The model under review builds one solid part; all positions refer to its coordinate system, in mm. Give positions to 0.01 mm unless a question says otherwise; leave off trailing zeros. Loops run counter-clockwise (first coordinate to the right, second up) from the corner with the lowest first, then second, coordinate; pieces in that order, holes last. Notation, with made-up numbers: (-2.75, 56) -> (31.25, 56) arc R21 ccw to (31.25, 95) -> close; hole circle Ø9 at (67.5, 59). An arc over 180 degrees is marked (long way). Write each question's results on one line, items separated by ' | '. Start each with the question number.
Q1. We need section B-B (z = -5.75). Write out the cut boundary in (x, y), plus the area to 3 significant figures.
Q2. Wall thickness on L1, parallel to X at y = 4.05, z = -6.75; L2, parallel to Z at x = -99, y = 1.45; L3, parallel to X at y = 3.4, z = -15.25: over which ranges is each line inside the solid? List them lowest first. Write a range as [from, to].
Q3. We need section A-A (y = 4.55). Write out the cut boundary in (x, z).
Q4. We need section D-D (z = -20). Write out the cut boundary in (x, y).
Q5. We need section C-C (x = -81). Write out the cut boundary in (y, z).
Q6. Insertion check: pin 1 Ø1.6 at (y, z) = (2.5, -7) entering from -X; pin 2 Ø1.6 at (x, y) = (85.5, 1.5) entering from +Z; pin 3 Ø2.5 at (y, z) = (3.5, -6) entering from +X. Each pin has a flat end and moves straight along its axis. Give the tip position at first contact, or say it passes through.
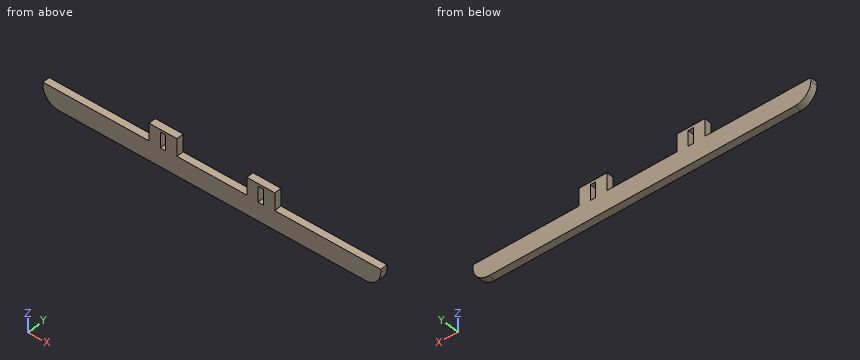
from build123d import *

# Parameters (mm, degrees)
SKETCH1_W             = 62
SKETCH1_H             = 12.7
BOSS_EXTRUDE1_DEPTH   = 5.38
SKETCH2_W             = 20.5
SKETCH2_H             = 5.38
CUT_EXTRUDE1_DEPTH    = 10.16
SKETCH3_W             = 4
SKETCH3_H             = 8.7
CUT_EXTRUDE2_DEPTH    = 5.38
SKETCH4_W             = 2.54
SKETCH4_H             = 5.38
BOSS_EXTRUDE2_DEPTH   = 59.22
SKETCH5_W             = 2.54
SKETCH5_H             = 5.38
BOSS_EXTRUDE3_DEPTH   = 11.5
BODY_MOVE_COPY3_ANGLE = 180
SKETCH6_W             = 21
SKETCH6_H             = 5.38
BOSS_EXTRUDE4_DEPTH   = 3
SKETCH7_W             = 21
SKETCH7_H             = 5.38
BOSS_EXTRUDE5_DEPTH   = 3
SKETCH8_W             = 4
SKETCH8_H             = 5.38
CUT_EXTRUDE3_DEPTH    = 3
SKETCH9_W             = 4
SKETCH9_H             = 5.38
CUT_EXTRUDE4_DEPTH    = 3
SKETCH11_W            = 253.94
SKETCH11_H            = 5.38
BOSS_EXTRUDE6_DEPTH   = 12
FILLET1_R             = 12


with BuildPart() as part:
    # Sketch1 → Boss-Extrude1 (new body)
    with BuildSketch(Plane(origin=(0, 0, 0), x_dir=(1, 0, 0), z_dir=(0, 1, 0))):
        with Locations((-31, 6.35)):
            Rectangle(SKETCH1_W, SKETCH1_H)
    extrude(amount=BOSS_EXTRUDE1_DEPTH)

    # Sketch2 → Cut-Extrude1 (cut)
    with BuildSketch(Plane.XY):
        with Locations((-51.75, 2.69)):
            Rectangle(SKETCH2_W, SKETCH2_H)
        with Locations((-10.25, 2.69)):
            Rectangle(SKETCH2_W, SKETCH2_H)
    extrude(amount=-CUT_EXTRUDE1_DEPTH, mode=Mode.SUBTRACT)

    # Sketch3 → Cut-Extrude2 (cut)
    with BuildSketch(Plane(origin=(0, 5.38, 0), x_dir=(1, 0, 0), z_dir=(0, 1, 0))):
        with Locations((-31, 6.35)):
            Rectangle(SKETCH3_W, SKETCH3_H)
    extrude(amount=-CUT_EXTRUDE2_DEPTH, mode=Mode.SUBTRACT)

    # Sketch4 → Boss-Extrude2 (add)
    with BuildSketch(Plane.ZY.offset(62)):
        with Locations((-11.43, 2.69)):
            Rectangle(SKETCH4_W, SKETCH4_H)
    extrude(amount=BOSS_EXTRUDE2_DEPTH)


with BuildPart() as body_2:
    # Body-Move/Copy1: copy of part
    add(part.part.moved(Location((0, 31.265873305, 0))))


with BuildPart() as part_1:
    add(part.part)

    # Sketch5 → Boss-Extrude3 (add)
    with BuildSketch(Plane(origin=(0, 0, 0), x_dir=(0, 0, -1), z_dir=(1, 0, 0))):
        with Locations((11.43, 2.69)):
            Rectangle(SKETCH5_W, SKETCH5_H)
    extrude(amount=BOSS_EXTRUDE3_DEPTH)


with BuildPart() as body_2_1:
    # Body-Move/Copy2: moved
    add(body_2.part.moved(Location((152.693560216, 0, 0))))


with BuildPart() as body_2_2:
    # Body-Move/Copy3: moved
    add(body_2_1.part.rotate(Axis((92.083560216, 33.955873305, 0), (0, 0, 1)), BODY_MOVE_COPY3_ANGLE))


with BuildPart() as body_2_3:
    # Body-Move/Copy4: read off the stored shape, not the designer's step
    # Body-Move/Copy4: moved
    add(body_2_2.part.moved(Location((-19.9735602, -31.2658733, 0))))

    # Combine1: union part
    add(part_1.part)

    # Sketch6 → Boss-Extrude4 (add)
    with BuildSketch(Plane.XY):
        with Locations((-31, 2.69)):
            Rectangle(SKETCH6_W, SKETCH6_H)
    extrude(amount=BOSS_EXTRUDE4_DEPTH)

    # Sketch7 → Boss-Extrude5 (add)
    with BuildSketch(Plane.XY):
        with Locations((42.5, 2.69)):
            Rectangle(SKETCH7_W, SKETCH7_H)
    extrude(amount=BOSS_EXTRUDE5_DEPTH)

    # Sketch8 → Cut-Extrude3 (cut)
    with BuildSketch(Plane(origin=(0, 0, -2), x_dir=(-1, 0, 0), z_dir=(0, 0, -1))):
        with Locations((31, 2.69)):
            Rectangle(SKETCH8_W, SKETCH8_H)
    extrude(amount=-CUT_EXTRUDE3_DEPTH, mode=Mode.SUBTRACT)

    # Sketch9 → Cut-Extrude4 (cut)
    with BuildSketch(Plane(origin=(0, 0, -2), x_dir=(-1, 0, 0), z_dir=(0, 0, -1))):
        with Locations((-42.5, 2.69)):
            Rectangle(SKETCH9_W, SKETCH9_H)
    extrude(amount=-CUT_EXTRUDE4_DEPTH, mode=Mode.SUBTRACT)

    # Sketch11 → Boss-Extrude6 (add)
    with BuildSketch(Plane(origin=(0, 0, -12.7), x_dir=(-1, 0, 0), z_dir=(0, 0, -1))):
        with Locations((-5.75, 2.69)):
            Rectangle(SKETCH11_W, SKETCH11_H)
    extrude(amount=BOSS_EXTRUDE6_DEPTH)

    # Fillet1
    fillet1_edges = [body_2_3.edges().sort_by_distance(p)[0] for p in [
        (132.72, 2.69, -24.7),
        (-121.22, 2.69, -24.7),
    ]]
    fillet(fillet1_edges, radius=FILLET1_R)


solid = body_2_3.part
Output:
1) outline: (-41.5, 0) -> (-33, 0) -> (-33, 5.38) -> (-41.5, 5.38) -> close; (-29, 0) -> (-20.5, 0) -> (-20.5, 5.38) -> (-29, 5.38) -> close; (32, 0) -> (40.5, 0) -> (40.5, 5.38) -> (32, 5.38) -> close; (44.5, 0) -> (53, 0) -> (53, 5.38) -> (44.5, 5.38) -> close | area: 183 mm2
2) L1: [-41.5, -33], [-29, -20.5], [32, 40.5], [44.5, 53] | L2: [-24.7, -10.16] | L3: [-120.95, 132.45]
3) outline: (-121.22, -12.7) arc R12 ccw to (-109.22, -24.7) -> (120.72, -24.7) arc R12 ccw to (132.72, -12.7) -> (132.72, -10.16) -> (53, -10.16) -> (53, 3) -> (32, 3) -> (32, -10.16) -> (-20.5, -10.16) -> (-20.5, 3) -> (-41.5, 3) -> (-41.5, -10.16) -> (-121.22, -10.16) -> close; hole (-33, -10.7) -> (-29, -10.7) -> (-29, 1) -> (-33, 1) -> close; hole (40.5, -10.7) -> (44.5, -10.7) -> (44.5, 1) -> (40.5, 1) -> close
4) outline: (-118.74, 0) -> (130.24, 0) -> (130.24, 5.38) -> (-118.74, 5.38) -> close
5) outline: (0, -24.7) -> (5.38, -24.7) -> (5.38, -10.16) -> (0, -10.16) -> close
6) pin 1: x = -41.5 | pin 2: z = -10.16 | pin 3: x = 53
